Check sheet for the modelled part. Datum: model origin and axes. Units: mm. Round coordinates to 2 decimals unless told otherwise and drop trailing zeros. Order: outer loops, then holes, each group sorted by start corner. A loop starts at its lowest first (then second) coordinate and runs counter-clockwise, first axis right, second up. Notation, with made-up numbers: (52, 31.25) -> (76, 31.25) arc R20 ccw to (76, 44.25) -> close; hole circle Ø10 at (22.5, 47.25). An arc over 180 degrees is marked (long way). Answer as CSV lines item,"result". Start each with the question number.
Autodesk Inventor part; units mm, degrees
ref_plane "Body2_1_XY" through (0, 0, 0) normal (0, 1, 0) x (1, 0, 0)
ref_plane "Body2_1_YZ" through (0, 0, 0) normal (1, 0, 0) x (0, 0, -1)
ref_plane "Body2_1_ZX" through (0, 0, 0) normal (0, 0, -1) x (0, 1, 0)
sketch "Sketch_1" plane through (0, 0, 0) normal (0, 0, 1) x (1, 0, 0)
  line L0 (0, -6.1) -> (0, 6.1)
  line L1 (0, 6.1) -> (1.64, 6.1)
  line L2 (1.64, 6.1) -> (1.64, -6.1)
  line L3 (1.64, -6.1) -> (0, -6.1)
  line L4 (0, -6.1) -> (0, 6.1)
revolve "Revolution1" add sketch "Sketch_1" angle 360 about axis through (0, -6.1, 0) along (0, -1, 0)
sketch "Sketch_7" plane through (0, 0, 0) normal (0, 0, 1) x (1, 0, 0)
  line L0 (0.82, 6.1) -> (2.46, 5.3353)
  line L1 (2.46, 5.3353) -> (2.46, 6.92)
  line L2 (2.46, 6.92) -> (0.82, 6.92)
  line L3 (0.82, 6.92) -> (0.82, 6.1)
extrude "Extrusion1" cut sketch "Sketch_7" along normal mid plane 3.28
sketch "Sketch_8" plane through (0, 0, 0) normal (0, 0, 1) x (1, 0, 0)
  line L0 (-2.46, 6.92) -> (-2.46, 5.3353)
  line L1 (-2.46, 5.3353) -> (-0.82, 6.1)
  line L2 (-0.82, 6.1) -> (-0.82, 6.92)
  line L3 (-0.82, 6.92) -> (-2.46, 6.92)
extrude "Extrusion2" cut sketch "Sketch_8" along normal mid plane 3.28
sketch "Sketch_9" plane through (0, 0, 0) normal (0, 0, 1) x (1, 0, 0)
  line L0 (0.82, -6.1) -> (0.82, -6.92)
  line L1 (0.82, -6.92) -> (2.46, -6.92)
  line L2 (2.46, -6.92) -> (2.46, -5.3353)
  line L3 (2.46, -5.3353) -> (0.82, -6.1)
extrude "Extrusion3" cut sketch "Sketch_9" along normal mid plane 3.28
sketch "Sketch_10" plane through (0, 0, 0) normal (0, 0, 1) x (1, 0, 0)
  line L0 (-2.46, -6.92) -> (-0.82, -6.92)
  line L1 (-0.82, -6.92) -> (-0.82, -6.1)
  line L2 (-0.82, -6.1) -> (-2.46, -5.3353)
  line L3 (-2.46, -5.3353) -> (-2.46, -6.92)
extrude "Extrusion4" cut sketch "Sketch_10" along normal mid plane 3.28
ref_plane "Body2_1_XY" through (0, 0, 0) normal (0, 1, 0) x (1, 0, 0)
ref_plane "Body2_1_YZ" through (0, 0, 0) normal (1, 0, 0) x (0, 0, -1)
ref_plane "Body2_1_ZX" through (0, 0, 0) normal (0, 0, -1) x (0, 1, 0)
ref_plane "for_pin_XY" through (0, -5.3803, 0) normal (1, 0, 0) x (0, 0, -1)
ref_plane "for_pin_YZ" through (0, -5.3803, 0) normal (0, 0, -1) x (0, 1, 0)
ref_plane "for_pin_ZX" through (0, -5.3803, 0) normal (0, 1, 0) x (1, 0, 0)
ref_plane "to_dummy_1_XY" through (0, 0, 0) normal (0, -1, 0) x (1, 0, 0)
ref_plane "to_dummy_1_YZ" through (0, 0, 0) normal (1, 0, 0) x (0, 0, 1)
ref_plane "to_dummy_1_ZX" through (0, 0, 0) normal (0, 0, 1) x (0, -1, 0)
properties part number "06B - 1 RP- Pin 1"
1) Section check C-C on z = -0.65. Record the cut outline in (x, y).
2) Material ranges on line 1 along Z through (x, y) = (-0.1, 1); line 2 along Z through (x, y) = (1, -1.5); line 3 along X through (y, z) = (-1, 1.15), recorded low to high.
3) Section check B-B on y = 0.5. Record the cut outline in (x, z).
4) Section check A-A on z = 0. Record the cut outline in (x, y), then the cut area to 3 significant figures.
Solutions:
1,outline,"(-1.51, -5.78) -> (-0.82, -6.1) -> (0.82, -6.1) -> (1.51, -5.78) -> (1.51, 5.78) -> (0.82, 6.1) -> (-0.82, 6.1) -> (-1.51, 5.78) -> close"
2,line 1,"z = -1.64 to 1.64"
2,line 2,"z = -1.3 to 1.3"
2,line 3,"x = -1.17 to 1.17"
3,outline,"circle Ø3.28 at (0, 0)"
4,outline,"(-1.64, -5.72) -> (-0.82, -6.1) -> (0.82, -6.1) -> (1.64, -5.72) -> (1.64, 5.72) -> (0.82, 6.1) -> (-0.82, 6.1) -> (-1.64, 5.72) -> close"
4,area,"39.4 mm^2"
